from build123d import *

# Parameters (mm, degrees)
AUFSATZ_LINEAR_AUSTRAGEN1_DEPTH = 10
AUFSATZ_LINEAR_AUSTRAGEN2_DEPTH = 8
VERRUNDUNG1_R                   = 2
SCHNITT_LINEAR_AUSTRAGEN1_REACH = 20
SKIZZE3_R                       = 10


with BuildPart() as part:
    # Skizze1 → Aufsatz-Linear austragen1 (new body)
    with BuildSketch(Plane(origin=(0, 0, 0), x_dir=(0, 0, -1), z_dir=(1, 0, 0))):
        with BuildLine():
            Line((-6.228450194, 19), (-13.106432709, 9.177222982))
            ThreePointArc((-13.106432709, 9.177222982), (0, -16), (13.106432709, 9.177222982))
            Line((13.106432709, 9.177222982), (6.228450194, 19))
            Line((6.228450194, 19), (-6.228450194, 19))
        make_face()
    extrude(amount=AUFSATZ_LINEAR_AUSTRAGEN1_DEPTH)

    # Skizze2 → Aufsatz-Linear austragen2 (add)
    with BuildSketch(Plane(origin=(10, 0, 0), x_dir=(0, 0, -1), z_dir=(1, 0, 0))):
        with BuildLine():
            Line((-12.287280664, 8.603646545), (-5.707883144, 18))
            Line((-5.707883144, 18), (5.707883144, 18))
            Line((5.707883144, 18), (12.287280664, 8.603646545))
            ThreePointArc((12.287280664, 8.603646545), (0, -15), (-12.287280664, 8.603646545))
        make_face()
    extrude(amount=AUFSATZ_LINEAR_AUSTRAGEN2_DEPTH)

    # Verrundung1
    verrundung1_edges = [part.edges().sort_by_distance(p)[0] for p in [
        (14, 18, -5.707883144),
        (14, 18, 5.707883144),
        (5, 19, -6.228450194),
        (5, 19, 6.228450194),
    ]]
    fillet(verrundung1_edges, radius=VERRUNDUNG1_R)

    # Skizze3 → Schnitt-Linear austragen1 (cut, up to next)
    with BuildSketch(Plane(origin=(18, 0, 0), x_dir=(0, 0, -1), z_dir=(1, 0, 0)), mode=Mode.PRIVATE) as schnitt_linear_austragen1_sk1:
        Circle(SKIZZE3_R)
    schnitt_linear_austragen1_tool1 = extrude(schnitt_linear_austragen1_sk1.sketch, amount=-SCHNITT_LINEAR_AUSTRAGEN1_REACH, mode=Mode.PRIVATE) & part.part
    add(schnitt_linear_austragen1_tool1.solids().sort_by_distance((18, 0, 0))[0], mode=Mode.SUBTRACT)


solid = part.part
The listing builds one solid part. Answer for the finished solid, in the listing's coordinates (mm). A direction names the side the tool comes from. Round coordinates to 2 decimals unless told otherwise and drop trailing zeros. Loops run counter-clockwise (first coordinate to the right, second up) from the corner with the lowest first, then second, coordinate; pieces in that order, holes last. Notation, with made-up numbers: M 64,-15 L 95,-15 A11 ccw 95,-10 Z; hole C -2.75,37.5 d8. An arc over 180 degrees is marked long. Return JSON: item names as keys, results as strings.
Q1. Find the intervals of material crossed by line 1 along Y through (x, z) = (4.75, 0); line 2 along X through (y, z) = (-10, 12); line 3 along Z through (x, y) = (12, 3.5), in increasing order. Write a range as from..to.
Results list:
{"line 1": "y = -16..-10, 10..19", "line 2": "x = 0..10", "line 3": "z = -14.59..-9.37, 9.37..14.59"}
Q2. Each of these flat-tipped pins is pushed along its axis until it touches: pin 1 Ø3 at (x, y) = (13.5, 13.5) entering from -Z; pin 2 Ø1.5 at (x, z) = (10, 7.5) entering from -Y; pin 3 Ø8 at (x, z) = (15.5, -7.5) entering from -Y; pin 4 Ø2 at (y, z) = (5.5, 4.5) entering from +X. Where does it stop, or does it pass through?
Results list:
{"pin 1": "stops at z = -9.91", "pin 2": "stops at y = -14.51", "pin 3": "stops at y = -14.59", "pin 4": "passes through"}
Q3. Find section D-D, the plane z = -11. Determine the outline of the cut face in (x, y).
Results list:
{"outline": "M 0,-11.62 L 10,-11.62 L 10,-10.2 L 18,-10.2 L 18,10.44 L 10,10.44 L 10,12.19 L 0,12.19 Z"}
Q4. Find section C-C, the plane x = 15.5. Determine the outline of the cut face in (y, z).
Results list:
{"outline": "M 8.6,-12.29 L 17.15,-6.31 A2 ccw 18,-4.67 L 18,4.67 A2 ccw 17.15,6.31 L 8.6,12.29 A15 ccw long Z; hole C 0,0 d20"}
Q5. The mould has two halves that part along Y. Classify faces 5 (the face through (9.13, -9.76, 2.17)), 6 (the face through (14.06, 17.78, 5.58)), 7 (the face through (14, -15, 0)): released by +Y, released by -Y, zero draft, split by the parting line, or undercut.
Results list:
{"face 5": "undercut", "face 6": "released by +Y", "face 7": "split by the parting line"}
Q6. Find section A-A, the plane y = 0. Determine the outline of the cut face in (x, z), plus the area to 3 significant figures.
Results list:
{"outline": "M 0,-16 L 10,-16 L 10,-15 L 18,-15 L 18,-10 L 0,-10 Z; M 0,10 L 18,10 L 18,15 L 10,15 L 10,16 L 0,16 Z", "area": "200 mm2"}
Q7. Which of the six approach directions +Z, -Z, +X, -X, +Y, -Y give full straight-line access (tool end or side, diameter ignored) to faces 1 (the face through (13.944, 12.816, 9.338)), 2 (the face through (13.94, 12.94, -9.25)), 3 (the face through (14, 18, 0)), 4 (the face through (10, 8, -13))?
Results list:
{"face 1": "+Z, +X, +Y", "face 2": "-Z, +X, +Y", "face 3": "+Z, -Z, +X, +Y", "face 4": "+X"}
Q8. Find section B-B, the plane z = 0. Determine the outline of the cut face in (x, y), plus the area to 3 significant figures.
Results list:
{"outline": "M 0,-16 L 10,-16 L 10,-15 L 18,-15 L 18,-10 L 0,-10 Z; M 0,10 L 18,10 L 18,18 L 10,18 L 10,19 L 0,19 Z", "area": "254 mm2"}
